```python
from build123d import *

# Parameters (mm, degrees)
SKETCH1_R           = 39
BOSS_EXTRUDE1_DEPTH = 4.5
SKETCH2_R           = 2.05
CUT_EXTRUDE1_DEPTH  = 4.5
SKETCH3_R           = 21
CUT_EXTRUDE2_DEPTH  = 4.5
SKETCH4_R           = 23.55
CUT_EXTRUDE3_DEPTH  = 2


with BuildPart() as part:
    # Sketch1 → Boss-Extrude1 (new body)
    with BuildSketch(Plane(origin=(0, 0, 0), x_dir=(1, 0, 0), z_dir=(0, 1, 0))):
        with Locations(Location((0, 0, 0), (0, 0, 270))):
            Circle(SKETCH1_R)
    extrude(amount=BOSS_EXTRUDE1_DEPTH)

    # Sketch2 → Cut-Extrude1 (cut)
    with BuildSketch(Plane(origin=(0, 4.5, 0), x_dir=(1, 0, 0), z_dir=(0, 1, 0))):
        with Locations(Location((31.75, 0, 0), (0, 0, 270))):
            Circle(SKETCH2_R)
        with Locations(Location((0, -31.75, 0), (0, 0, 270))):
            Circle(SKETCH2_R)
        with Locations(Location((-31.75, 0, 0), (0, 0, 270))):
            Circle(SKETCH2_R)
        with Locations(Location((0, 31.75, 0), (0, 0, 270))):
            Circle(SKETCH2_R)
    extrude(amount=-CUT_EXTRUDE1_DEPTH, mode=Mode.SUBTRACT)

    # Sketch3 → Cut-Extrude2 (cut)
    with BuildSketch(Plane(origin=(0, 4.5, 0), x_dir=(1, 0, 0), z_dir=(0, 1, 0))):
        with Locations(Location((0, 0, 0), (0, 0, 270))):
            Circle(SKETCH3_R)
    extrude(amount=-CUT_EXTRUDE2_DEPTH, mode=Mode.SUBTRACT)

    # Sketch4 → Cut-Extrude3 (cut)
    with BuildSketch(Plane(origin=(0, 4.5, 0), x_dir=(1, 0, 0), z_dir=(0, 1, 0))):
        with Locations(Location((0, 0, 0), (0, 0, 270))):
            Circle(SKETCH4_R)
    extrude(amount=-CUT_EXTRUDE3_DEPTH, mode=Mode.SUBTRACT)


solid = part.part
```
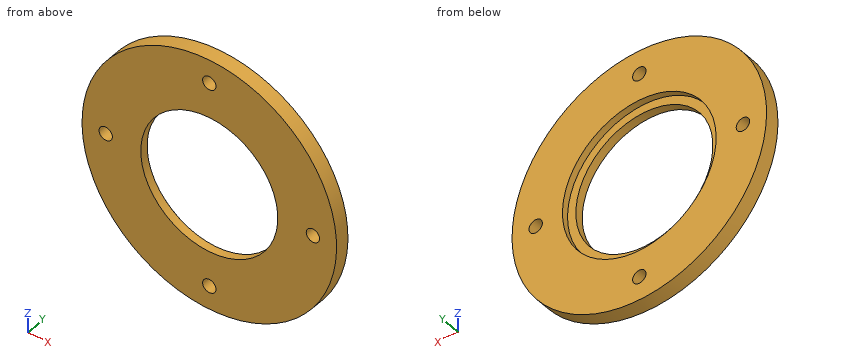
Work out the finished part from the listing and answer in its coordinate system (mm). Coordinates: 2 decimals unless noted, no trailing zeros. Loops run counter-clockwise (first coordinate to the right, second up) from the corner with the lowest first, then second, coordinate; pieces in that order, holes last. Notation, with made-up numbers: M 81.25,34.25 L 104.25,34.25 A28 cw 104.25,64.25 Z; hole C 28.5,26.25 d4. An arc over 180 degrees is marked long. Use CSV: the item, a comma, the result in double quotes. Start each with the question number.
(1) Given pin 1 Ø2 at (x, y) = (-1.5, 3.5) entering from -Z, flat-ended and moving along its own axis, determine where the tip first touches the part or whether it passes through.
(2) Consider line 1 (X direction, y = 1.65, z = 0); line 2 (X direction, y = 2.8, z = 0); line 3 (Y direction, x = -7, z = -21.5). Determine where each line is inside the solid, lowest interval first.
(3) Find section B-B, the plane z = 0. Give the vertices of the cut face in (x, y), then the cut area to 3 significant figures.
(4) Find section A-A, the plane x = 0. Give the vertices of the cut face in (y, z).
(5) Find section D-D, the plane y = 1.5. Give the vertices of the cut face in (x, z).
(6) Find section C-C, the plane x = 14. Give the vertices of the cut face in (y, z), then the cut area to 3 significant figures.
Recorded:
1,pin 1,"stops at z = -39"
2,line 1,"x = -39 to -33.8, -29.7 to -21, 21 to 29.7, 33.8 to 39"
2,line 2,"x = -39 to -33.8, -29.7 to -23.55, 23.55 to 29.7, 33.8 to 39"
2,line 3,"y = 0 to 2.5"
3,outline,"M -39,0 L -33.8,0 L -33.8,4.5 L -39,4.5 Z; M -29.7,0 L -21,0 L -21,2.5 L -23.55,2.5 L -23.55,4.5 L -29.7,4.5 Z; M 21,0 L 29.7,0 L 29.7,4.5 L 23.55,4.5 L 23.55,2.5 L 21,2.5 Z; M 33.8,0 L 39,0 L 39,4.5 L 33.8,4.5 Z"
3,area,"115 mm^2"
4,outline,"M 0,-39 L 4.5,-39 L 4.5,-33.8 L 0,-33.8 Z; M 0,-29.7 L 4.5,-29.7 L 4.5,-23.55 L 2.5,-23.55 L 2.5,-21 L 0,-21 Z; M 0,21 L 2.5,21 L 2.5,23.55 L 4.5,23.55 L 4.5,29.7 L 0,29.7 Z; M 0,33.8 L 4.5,33.8 L 4.5,39 L 0,39 Z"
5,outline,"C 0,0 d78; hole C -31.75,0 d4.1; hole C 0,0 d42; hole C 0,-31.75 d4.1; hole C 0,31.75 d4.1; hole C 31.75,0 d4.1"
6,outline,"M 0,-36.4 L 4.5,-36.4 L 4.5,-18.94 L 2.5,-18.94 L 2.5,-15.65 L 0,-15.65 Z; M 0,15.65 L 2.5,15.65 L 2.5,18.94 L 4.5,18.94 L 4.5,36.4 L 0,36.4 Z"
6,area,"174 mm^2"
